Drawing for the job (mm, zero at the part's lowest x, y, z). A direction names the side the tool comes from. Give positions to 0.01 mm unless a question says otherwise; leave off trailing zeros. Loops run counter-clockwise (first coordinate to the right, second up) from the corner with the lowest first, then second, coordinate; pieces in that order, holes last. Notation, with made-up numbers: M -24.5,-27 L 14.5,-27 A26 ccw 14.5,-10 Z; hole C 26.5,-17.5 d5. An arc over 180 degrees is marked long. Use CSV: the item, a comma, the result in double quotes. Start each with the question number.
(1) Slice it at D-D on z = 30. List the corners of the cut face in (x, y).
(2) Wall check: line 1 along Z through (x, y) = (6, 4.25); line 2 along X through (y, z) = (3.5, 27.5); line 3 along X through (y, z) = (3.5, 35). Give the ranges that are in metal, low to high. Write a range as from..to.
(3) Slice it at A-A on x = 64. List the corners of the cut face in (y, z), and give its area (3 significant figures).
(4) Two-plate mould, pull along Z, no slides. Class the marked faces 1, 2 and 3: pulls with the +Z half, pulls with the -Z half, needs draft (parallel to the pull), parting line crosses it, or undercut.
(5) Flat gauge pins, fed straight in: P1, Ø10, axis at x = 37, z = 26.5, coming from the +Y side; P2, Ø5.5, axis at x = 6, z = 8, coming from the +Y side; P3, Ø1.5, axis at x = 49, y = 2.5, coming from the +Z side; P4, Ø1, axis at x = 49, y = 4.5, coming from the +Z side. Where does each tip first touch, or does it go through?
(6) Slice it at C-C on y = 3.5. List the corners of the cut face in (x, z), and give its area (3 significant figures).
(7) Tool access for the marked faces 4 and 5: list every direction of +Z, -Z, +X, -X, +Y, -Y with a clear straight run to the whole face (end or side of a thin tool).
(8) Slice it at B-B on z = 8. List the corners of the cut face in (x, y).
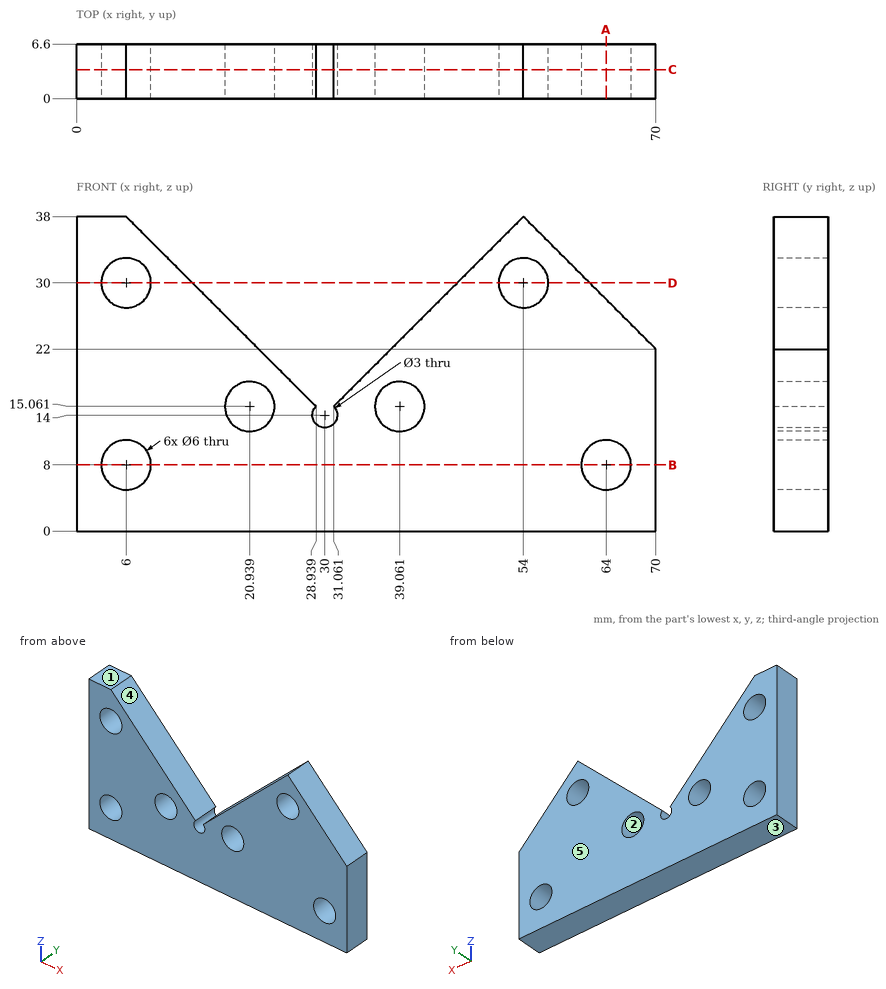
Reply:
1,outline,"M 0,0 L 3,0 L 3,6.6 L 0,6.6 Z; M 9,0 L 14,0 L 14,6.6 L 9,6.6 Z; M 46,0 L 51,0 L 51,6.6 L 46,6.6 Z; M 57,0 L 62,0 L 62,6.6 L 57,6.6 Z"
2,line 1,"z = 0..5, 11..27, 33..38"
2,line 2,"x = 0..4.34, 7.66..16.5, 43.5..52.34, 55.66..64.5"
2,line 3,"x = 0..9, 51..57"
3,outline,"M 0,0 L 6.6,0 L 6.6,5 L 0,5 Z; M 0,11 L 6.6,11 L 6.6,28 L 0,28 Z"
3,area,"145 mm^2"
4,face 1,"pulls with the +Z half"
4,face 2,"undercut"
4,face 3,"pulls with the -Z half"
5,P1,"stops at y = 6.6"
5,P2,"passes through"
5,P3,"stops at z = 33.75"
5,P4,"stops at z = 33.5"
6,outline,"M 0,0 L 70,0 L 70,22 L 54,38 L 31.06,15.06 A1.5 cw long 28.94,15.06 L 6,38 L 0,38 Z; hole C 6,8 d6; hole C 6,30 d6; hole C 20.94,15.06 d6; hole C 39.06,15.06 d6; hole C 54,30 d6; hole C 64,8 d6"
6,area,"1,780 mm^2"
7,face 4,"+Z, +Y, -Y"
7,face 5,"+Z, -Z, +X, -X, +Y"
8,outline,"M 0,0 L 3,0 L 3,6.6 L 0,6.6 Z; M 9,0 L 61,0 L 61,6.6 L 9,6.6 Z; M 67,0 L 70,0 L 70,6.6 L 67,6.6 Z"
